from build123d import *

# Parameters (mm, degrees)
SKETCH1_R           = 25.4
SKETCH1_R_2         = 6.35
BOSS_EXTRUDE1_DEPTH = 9.525
SKETCH2_R           = 12.7
SKETCH2_R_2         = 6.35
BOSS_EXTRUDE2_DEPTH = 39.37
SKETCH3_R           = 22.225
SKETCH3_R_2         = 12.7
BOSS_EXTRUDE3_DEPTH = 6.35


with BuildPart() as part:
    # Sketch1 → Boss-Extrude1 (new body)
    with BuildSketch(Plane.XY):
        with BuildLine():
            ThreePointArc((25.293941551, -2.318732586), (0, -25.4), (-25.293941551, -2.318732586))
            Line((-25.293941551, -2.318732586), (-12.7, -139.7))
            Line((-12.7, -139.7), (12.7, -139.7))
            Line((12.7, -139.7), (25.293941551, -2.318732586))
        make_face()
        Circle(SKETCH1_R)
        Circle(SKETCH1_R_2, mode=Mode.SUBTRACT)
    boss_extrude1 = extrude(amount=BOSS_EXTRUDE1_DEPTH)

    # Sketch2 → Boss-Extrude2 (add)
    with BuildSketch(Plane.XY.offset(9.525)):
        Circle(SKETCH2_R)
        Circle(SKETCH2_R_2, mode=Mode.SUBTRACT)
    extrude(amount=BOSS_EXTRUDE2_DEPTH)

    # Mirror2: Boss-Extrude1 across plane
    add(boss_extrude1.mirror(Plane(origin=(0, 0, 29.21), x_dir=(1, 0, 0), z_dir=(0, 0, -1))))

    # Sketch3 → Boss-Extrude3 (add)
    with BuildSketch(Plane(origin=(0, 0, 39.878), x_dir=(-1, 0, 0), z_dir=(0, 0, -1))):
        Circle(SKETCH3_R)
        Circle(SKETCH3_R_2, mode=Mode.SUBTRACT)
    extrude(amount=-BOSS_EXTRUDE3_DEPTH)


solid = part.part
The listing builds one solid part. Answer for the finished solid, in the listing's coordinates (mm). A direction names the side the tool comes from. Round coordinates to 2 decimals unless told otherwise and drop trailing zeros. Write each loop counter-clockwise with the first axis right and the second up, starting at its lowest first coordinate (ties: lowest second). Pieces come first, ordered by that corner, then holes. Notation, with made-up numbers: M 71,-30 L 102,-30 A10 ccw 102,-23 Z; hole C 36.25,18 d4. An arc over 180 degrees is marked long. Write each question's results on one line, items separated by ' | '. Start each with the question number.
Item 1: Find section B-B on x = 0. Write down the section's boundary in (y, z) (3 decimals), and give its area (3 significant figures).
Item 2: Given pin 1 Ø2 at (x, z) = (-3, 31) entering from -Y; pin 2 Ø12 at (x, z) = (17.5, 29.5) entering from -Y; pin 3 Ø8 at (x, z) = (-7.5, 40.5) entering from -Y; pin 4 Ø1.5 at (x, z) = (-15.5, 11) entering from +Y, each flat-ended and moving along its own axis, determine where each tip first touches the part or whether it passes through.
Item 3: Find section A-A on y = 0. Write down the section's boundary in (x, z) (3 decimals).
Item 4: The mould has two halves that part along Z. Classify faces 3 (the flat face through (0, -139.7, 5)), 4 (the flat face through (0, -56, 58.42)), 5 (the cylindrical face through (-2.75, -12.4, 24.49)), 6 (the flat face through (-10, -10, 39.878)): +Z half, -Z half, draft (parallel to the pull), parting line (faces both ways), or undercut.
Item 5: Which of the six approach directions +Z, -Z, +X, -X, +Y, -Y give full straight-line access (tool end or side, diameter ignored) to faces 1 (the cylindrical face through (-21.199, 6.676, 43.009)), 2 (the flat face through (0, -139.7, 54))?
Item 6: Straight lines are drawn through the part: probe 1 along Z at (x, y) = (-9.5, -71.5) (3 decimals); probe 2 along Y at (x, z) = (0, 35); probe 3 along Z at (x, y) = (18.5, -3.5) (3 decimals). For each, find the intervals that lie inside material, in ascending order.
Item 7: Find section D-D on z = 37. Write down the section's boundary in (x, y).
Item 8: Find section C-C on x = -19.5. Write down the section's boundary in (y, z) (3 decimals).
Answer block:
1) outline: M -139.7,0 L -6.35,0 L -6.35,58.42 L -139.7,58.42 L -139.7,48.895 L -12.7,48.895 L -12.7,46.228 L -22.225,46.228 L -22.225,39.878 L -12.7,39.878 L -12.7,9.525 L -139.7,9.525 Z; M 6.35,0 L 25.4,0 L 25.4,9.525 L 12.7,9.525 L 12.7,39.878 L 22.225,39.878 L 22.225,46.228 L 12.7,46.228 L 12.7,48.895 L 25.4,48.895 L 25.4,58.42 L 6.35,58.42 Z | area: 3,520 mm²
2) pin 1: stops at y = -12.54 | pin 2: stops at y = -5.39 | pin 3: stops at y = -21.95 | pin 4: passes through
3) outline: M -25.4,0 L -6.35,0 L -6.35,58.42 L -25.4,58.42 L -25.4,48.895 L -12.7,48.895 L -12.7,46.228 L -22.225,46.228 L -22.225,39.878 L -12.7,39.878 L -12.7,9.525 L -25.4,9.525 Z; M 6.35,0 L 25.4,0 L 25.4,9.525 L 12.7,9.525 L 12.7,39.878 L 22.225,39.878 L 22.225,46.228 L 12.7,46.228 L 12.7,48.895 L 25.4,48.895 L 25.4,58.42 L 6.35,58.42 Z
4) face 3: draft | face 4: +Z half | face 5: undercut | face 6: undercut
5) face 1: none | face 2: +Z, -Z, +X, -X, -Y
6) probe 1: z = 0 to 9.525, 48.895 to 58.42 | probe 2: y = -12.7 to -6.35, 6.35 to 12.7 | probe 3: z = 0 to 9.525, 39.878 to 46.228, 48.895 to 58.42
7) outline: C 0,0 d25.4; hole C 0,0 d12.7
8) outline: M -65.522,0 L 16.276,0 L 16.276,9.525 L -65.522,9.525 Z; M -65.522,48.895 L 16.276,48.895 L 16.276,58.42 L -65.522,58.42 Z; M -10.663,39.878 L 10.663,39.878 L 10.663,46.228 L -10.663,46.228 Z
